Source: CAD feature listing. Evaluate the final solid. Frame: model axes, mm. Give positions to 0.01 mm unless a question says otherwise; leave off trailing zeros. Write each loop counter-clockwise with the first axis right and the second up, starting at its lowest first coordinate (ties: lowest second). Pieces come first, ordered by that corner, then holes. Notation, with made-up numbers: (-5, 8) -> (37, 8) arc R21 cw to (37, 29) -> close; hole circle Ø5 at (-3, 25.5). An arc over 180 degrees is marked (long way). Answer as a JSON object with one key per item and string values. Group by question number.
Item 1: Section query B-B on z = 10.5. Return the cut outline in (x, y) (3 decimals), plus the area to 3 significant figures.
Item 2: Section query D-D on x = -1.75. Return the cut outline in (y, z).
Item 3: Section query A-A on x = 0. Return the cut outline in (y, z), plus the area to 3 significant figures.
Item 4: Section query C-C on y = 7.5. Return the cut outline in (x, z), plus the area to 3 significant figures.
Item 5: Ray query, probe 1 along Y at (x, z) = (0, 1.55); probe 2 along Y at (x, z) = (0, 15.75); probe 3 along X at (y, z) = (18, 4.75). Return the intervals inside material, ascending. Write a range as from..to.
Item 6: First-contact query: pin 1 Ø3 at (x, y) = (0, -10.15) entering from -Z; pin 2 Ø10 at (y, z) = (-4, 10.5) entering from +X; pin 3 Ø1.5 at (x, y) = (-1, -2.5) entering from +Z; pin 4 Ø2 at (x, z) = (1.5, 10.5) entering from +Y. Flat tips, straight axial feed; report the tip coordinate or a pass-through.
Item 7: Pull-direction query (Y, two-part tool) for faces 1 (the face through (0.055, -12.646, 1.972)), 2 (the face through (-0.179, -8.784, 1.972)), 3 (the face through (0.542, 20.293, 9.86)), 4 (the face through (0, 3, 4)); classes: pulls with the +Y half, pulls with the -Y half, needs draft (parallel to the pull), parting line crosses it, or undercut.
from build123d import *

# Parameters (mm, degrees)
SKETCH1_R           = 1.375
BOSS_EXTRUDE3_DEPTH = 4
SKETCH1_6_R         = 1.375
BOSS_EXTRUDE4_DEPTH = 20


with BuildPart() as part:
    # Sketch1 → Boss-Extrude3 (new body)
    with BuildSketch(Plane.XY):
        with BuildLine():
            Line((-2.5, -10.147058824), (-2.5, 17.852941176))
            ThreePointArc((-2.5, 17.852941176), (0, 15.352941176), (2.5, 17.852941176))
            Line((2.5, 17.852941176), (2.5, -10.147058824))
            ThreePointArc((2.5, -10.147058824), (0, -12.647058824), (-2.5, -10.147058824))
        make_face()
        with Locations((0, -10.147058824)):
            Circle(SKETCH1_R, mode=Mode.SUBTRACT)
    extrude(amount=BOSS_EXTRUDE3_DEPTH)

    # Sketch1_6 → Boss-Extrude4 (add)
    with BuildSketch(Plane.XY):
        with BuildLine():
            ThreePointArc((2.5, 17.852941176), (0, 20.352941176), (-2.5, 17.852941176))
            ThreePointArc((-2.5, 17.852941176), (0, 15.352941176), (2.5, 17.852941176))
        make_face()
        with Locations((0, 17.852941176)):
            Circle(SKETCH1_6_R, mode=Mode.SUBTRACT)
    extrude(amount=BOSS_EXTRUDE4_DEPTH)


solid = part.part
Worked answers:
{
 "1": {"outline": "circle Ø5 at (0, 17.853); hole circle Ø2.75 at (0, 17.853)", "area": "13.7 mm^2"},
 "2": {"outline": "(-11.93, 0) -> (19.64, 0) -> (19.64, 20) -> (16.07, 20) -> (16.07, 4) -> (-11.93, 4) -> close"},
 "3": {"outline": "(-12.65, 0) -> (-11.52, 0) -> (-11.52, 4) -> (-12.65, 4) -> close; (-8.77, 0) -> (16.48, 0) -> (16.48, 20) -> (15.35, 20) -> (15.35, 4) -> (-8.77, 4) -> close; (19.23, 0) -> (20.35, 0) -> (20.35, 20) -> (19.23, 20) -> close", "area": "146 mm^2"},
 "4": {"outline": "(-2.5, 0) -> (2.5, 0) -> (2.5, 4) -> (-2.5, 4) -> close", "area": "20.0 mm^2"},
 "5": {"probe 1": "-12.65..-11.52, -8.77..16.48, 19.23..20.35", "probe 2": "15.35..16.48, 19.23..20.35", "probe 3": "-2.5..-1.37, 1.37..2.5"},
 "6": {"pin 1": "z = 0", "pin 2": "through", "pin 3": "z = 4", "pin 4": "y = 20.3"},
 "7": {"face 1": "pulls with the -Y half", "face 2": "undercut", "face 3": "parting line crosses it", "face 4": "needs draft"}
}
